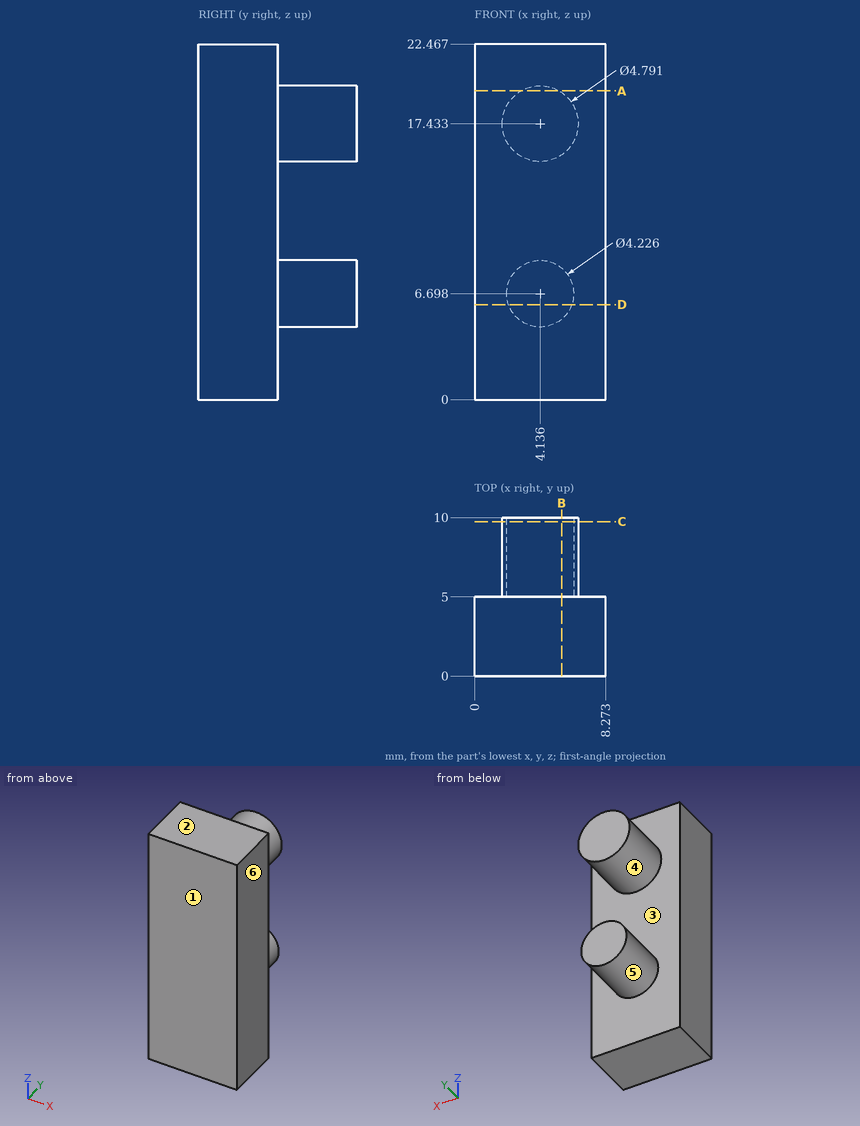
Could you check a few things on this drawing? It's one solid part, dimensions in mm from its lowest x, y, z. A direction names the side the tool comes from. Coordinates: 2 decimals unless noted, no trailing zeros. Write each loop counter-clockwise with the first axis right and the second up, starting at its lowest first coordinate (ties: lowest second). Pieces come first, ordered by that corner, then holes.
1) If we section it at D-D (z = 6): List the corners of the cut face in (x, y) for me.
Filled in:
outline: (0, 0) - (8.27, 0) - (8.27, 5) - (6.13, 5) - (6.13, 10) - (2.14, 10) - (2.14, 5) - (0, 5) - close
2) If we section it at B-B (x = 5.5): List the corners of the cut face in (y, z) for me.
Filled in:
outline: (0, 0) - (5, 0) - (5, 5.08) - (10, 5.08) - (10, 8.31) - (5, 8.31) - (5, 15.46) - (10, 15.46) - (10, 19.4) - (5, 19.4) - (5, 22.47) - (0, 22.47) - close
3) If we section it at C-C (y = 9.75): List the corners of the cut face in (x, z) for me (1 decimal).
Filled in:
outline: circle Ø4.8 at (4.1, 17.4); circle Ø4.2 at (4.1, 6.7)
4) If I drill on line 1 (Y direction, x = 0.75, z = 6.5); line 2 (Z direction, x = 6, y = 7.75) (1 decimal); line 3 (Z direction, x = 3, y = 7.25) (1 decimal), over which ranges is the centre line in solid material (lowest first)?
Filled in:
line 1: y = 0 to 5
line 2: z = 5.7 to 7.7, 15.9 to 18.9
line 3: z = 4.9 to 8.5, 15.3 to 19.5
5) Which directions (+Z, -Z, +X, -X, +Y, -Y) give clear straight access to the entire face, cutting with the end or side of a thin tool? Please do the marked faces 5 and 6.
Filled in:
face 5: +Y
face 6: +Z, -Z, +X, +Y, -Y
6) Thinking about a two-plate mould opening in Z: for the marked faces 1, 2, 3 and 4, which applies, +Z half, -Z half, draft (parallel to the pull), parting line (faces both ways), or undercut?
Filled in:
face 1: draft
face 2: +Z half
face 3: undercut
face 4: undercut
7) If we section it at A-A (z = 19.5): List the corners of the cut face in (x, y) for me.
Filled in:
outline: (0, 0) - (8.27, 0) - (8.27, 5) - (5.35, 5) - (5.35, 10) - (2.93, 10) - (2.93, 5) - (0, 5) - close
